from build123d import *

# Parameters (mm, degrees)
SKETCH_1_W                   = 73
SKETCH_1_H                   = 100
EXTRUDE_1_DEPTH              = 10
HOLE_WIZARD_M5_1_D           = 5.8
HOLE_WIZARD_M5_1_CBORE_D     = 10
HOLE_WIZARD_M5_1_CBORE_DEPTH = 5
HOLE_WIZARD_M5_1_2_D         = 4.2
HOLE_WIZARD_M5_1_2_DEPTH     = 12.4
HOLE_WIZARD_M5_1_2_TIP       = 1.2618073
SKETCH_6_W                   = 23
SKETCH_6_H                   = 35
CUT_EXTRUDE_1_DEPTH          = 125.213525834


with BuildPart() as part:
    # 草图1 → 凸台-拉伸1 (new body)
    with BuildSketch(Plane.XY):
        with Locations((36.5, 50)):
            Rectangle(SKETCH_1_W, SKETCH_1_H)
    extrude(amount=EXTRUDE_1_DEPTH)

    # Hole Wizard M5 _1 (through all)
    with Locations(Plane(origin=(0, 0, 0), x_dir=(-1, 0, 0), z_dir=(0, 0, -1))):
        with Locations((-10, 80), (-43, 94), (-10, 45)):
            CounterBoreHole(HOLE_WIZARD_M5_1_D / 2, HOLE_WIZARD_M5_1_CBORE_D / 2, HOLE_WIZARD_M5_1_CBORE_DEPTH)

    # Hole Wizard M5 _1 2
    with Locations(Plane(origin=(73, 0, 0), x_dir=(0, 0, -1), z_dir=(1, 0, 0))):
        with Locations((-5, 80), (-5, 45)):
            Hole(HOLE_WIZARD_M5_1_2_D / 2, depth=HOLE_WIZARD_M5_1_2_DEPTH)
            with Locations((0, 0, -(HOLE_WIZARD_M5_1_2_DEPTH + HOLE_WIZARD_M5_1_2_TIP / 2))):  # 118° drill point
                Cone(0, HOLE_WIZARD_M5_1_2_D / 2, HOLE_WIZARD_M5_1_2_TIP, mode=Mode.SUBTRACT)

    # 草图6 → 切除-拉伸1 (cut, through all)
    with BuildSketch(Plane(origin=(0, 0, 0), x_dir=(-1, 0, 0), z_dir=(0, 0, -1))):
        with Locations((-11.5, 17.5)):
            Rectangle(SKETCH_6_W, SKETCH_6_H)
    extrude(amount=-CUT_EXTRUDE_1_DEPTH, mode=Mode.SUBTRACT)


solid = part.part
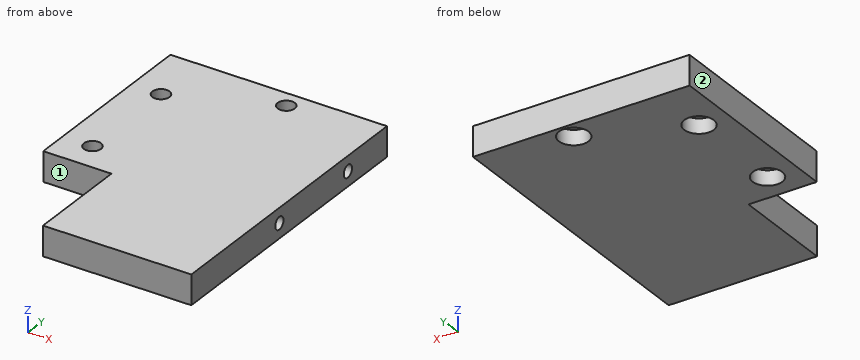
Read the model definition and answer for the solid it produces. Units are mm, in the model's axes. Face numbers are marked on the shaded views. A direction names the side the tool comes from. Coordinates: 2 decimals unless noted, no trailing zeros. Loops run counter-clockwise (first coordinate to the right, second up) from the corner with the lowest first, then second, coordinate; pieces in that order, holes last.
Q1. Consider probe 1 along Y at (x, z) = (10, 7.8); probe 2 along Y at (x, z) = (10, 2.45); probe 3 along Y at (x, z) = (43, 2.85). Determine where each line is inside the solid, lowest interval first.
Q2. The part is cut by section D-D on y = 30.5. Write down the section's boundary in (x, z), and give its area (3 significant figures).
Q3. The part is cut by section B-B on z = 8.5. Write down the section's boundary in (x, y).
Q4. Which of the six approach directions +Z, -Z, +X, -X, +Y, -Y give full straight-line access (tool end or side, diameter ignored) to the marked faces 1 and 2?
Q5. The part is cut by section C-C on x = 10. Write down the section's boundary in (y, z), and give its area (3 significant figures).
Q6. Each of these flat-tipped pins is pushed along its axis until it touches: pin 1 Ø5 at (x, y) = (9, 81) entering from -Z; pin 2 Ø3 at (x, z) = (14.5, 7) entering from -Y. Where does it stop, or does it pass through?
Q7. The part is cut by section A-A on x = 43. Write down the section's boundary in (y, z), and give its area (3 significant figures).
Results below:
1. probe 1: y = 35 to 42.1, 47.9 to 77.1, 82.9 to 100
1. probe 2: y = 35 to 40, 50 to 75, 85 to 100
1. probe 3: y = 0 to 89, 99 to 100
2. outline: (23, 0) - (73, 0) - (73, 10) - (23, 10) - close
2. area: 500 mm2
3. outline: (0, 35) - (23, 35) - (23, 0) - (73, 0) - (73, 100) - (0, 100) - close; hole circle Ø5.8 at (10, 45); hole circle Ø5.8 at (10, 80); hole circle Ø5.8 at (43, 94)
4. face 1: +Z, -Z, -X, -Y
4. face 2: +Z, -Z, -X, +Y, -Y
5. outline: (35, 0) - (40, 0) - (40, 5) - (42.1, 5) - (42.1, 10) - (35, 10) - close; (47.9, 5) - (50, 5) - (50, 0) - (75, 0) - (75, 5) - (77.1, 5) - (77.1, 10) - (47.9, 10) - close; (82.9, 5) - (85, 5) - (85, 0) - (100, 0) - (100, 10) - (82.9, 10) - close
5. area: 492 mm2
6. pin 1: stops at z = 5
6. pin 2: stops at y = 35
7. outline: (0, 0) - (89, 0) - (89, 5) - (91.1, 5) - (91.1, 10) - (0, 10) - close; (96.9, 5) - (99, 5) - (99, 0) - (100, 0) - (100, 10) - (96.9, 10) - close
7. area: 921 mm2
